Geometry check sheet. Reference: the model listing, model coordinates, mm. A direction names the side the tool comes from. Round coordinates to 2 decimals unless told otherwise and drop trailing zeros. Order: outer loops, then holes, each group sorted by start corner. A loop starts at its lowest first (then second) coordinate and runs counter-clockwise, first axis right, second up. Notation, with made-up numbers: (-6.5, 13.25) - (9.5, 13.25) arc R16 cw to (9.5, 27.25) - close; hole circle Ø4 at (53, 61). An arc over 180 degrees is marked (long way). Use a Markdown table: item, result. Add a question column.
(1) Section check D-D on z = 16. Record the boundary of the cut face in (x, y), then the cut area to 3 significant figures.
(2) Mould release check, pull along X, two halves, no side actions. Record for faces 1 (the face through (0.061, -17.445, 87.468)), 2 (the face through (0, 0, 126)), 3 (the face through (-10.88, -11.27, 87.47)): released by +X, released by -X, zero draft, split by the parting line, or undercut.
(3) Thickness scan on line 1 along X through (y, z) = (10.5, 53); line 2 along X through (y, z) = (14, 100); line 3 along Y through (x, z) = (-14.5, 103.5). Record the ranges inside material, lowest first. Write a range as [from, to].
(4) Section check B-B on y = 0. Record the boundary of the cut face in (x, z) (3 decimals).
(5) Gauge pin test, flat ends, axial feed: P1, Ø6, axis at y = 12, z = 88, coming from the -X side; P2, Ø12, axis at x = 9, z = 33, coming from the +Y side; P3, Ø10, axis at y = 1.5, z = 24.5, coming from the +X side. Record the tip position at first contact, or that the pin passes through.
(6) Access from +Z, -Z, +X, -X, +Y, -Y to the whole of each face (thin tool, end or side, straight path). Record for faces 4 (the face through (-10.922, 11.294, 87.468)), 5 (the face through (15.198, -3.786, 87.468)), 6 (the face through (-5, -12, 50)).
(7) Section check A-A on x = 0. Record the boundary of the cut face in (y, z) (3 decimals).
(8) Section check C-C on z = 59.5. Record the boundary of the cut face in (x, y) (3 decimals), then the cut area to 3 significant figures.
```python
from build123d import *

# Parameters (mm, degrees)
SKETCH1_R           = 12.5
BOSS_EXTRUDE1_DEPTH = 50
BOSS_EXTRUDE2_DEPTH = 76


with BuildPart() as part:
    # Sketch1 → Boss-Extrude1 (new body)
    with BuildSketch(Plane.XY):
        Circle(SKETCH1_R)
    extrude(amount=BOSS_EXTRUDE1_DEPTH)

    # Sketch2 → Boss-Extrude2 (add)
    with BuildSketch(Plane.XY.offset(50)):
        with BuildLine():
            Line((9.322615937, 10.370721146), (12.477254481, 12.192052559))
            ThreePointArc((12.477254481, 12.192052559), (15.107813169, 8.7225), (16.797254481, 4.709593071))
            Line((16.797254481, 4.709593071), (13.642615937, 2.888261658))
            ThreePointArc((13.642615937, 2.888261658), (13.945, 0), (13.642615937, -2.888261658))
            Line((13.642615937, -2.888261658), (16.797254481, -4.709593071))
            ThreePointArc((16.797254481, -4.709593071), (15.107813169, -8.7225), (12.477254481, -12.192052559))
            Line((12.477254481, -12.192052559), (9.322615937, -10.370721146))
            ThreePointArc((9.322615937, -10.370721146), (6.9725, -12.076724256), (4.32, -13.258982804))
            Line((4.32, -13.258982804), (4.32, -16.90164563))
            ThreePointArc((4.32, -16.90164563), (0, -17.445), (-4.32, -16.90164563))
            Line((-4.32, -16.90164563), (-4.32, -13.258982804))
            ThreePointArc((-4.32, -13.258982804), (-6.9725, -12.076724256), (-9.322615937, -10.370721146))
            Line((-9.322615937, -10.370721146), (-12.477254481, -12.192052559))
            ThreePointArc((-12.477254481, -12.192052559), (-15.107813169, -8.7225), (-16.797254481, -4.709593071))
            Line((-16.797254481, -4.709593071), (-13.642615937, -2.888261658))
            ThreePointArc((-13.642615937, -2.888261658), (-13.945, 0), (-13.642615937, 2.888261658))
            Line((-13.642615937, 2.888261658), (-16.797254481, 4.709593071))
            ThreePointArc((-16.797254481, 4.709593071), (-15.107813169, 8.7225), (-12.477254481, 12.192052559))
            Line((-12.477254481, 12.192052559), (-9.322615937, 10.370721146))
            ThreePointArc((-9.322615937, 10.370721146), (-6.9725, 12.076724256), (-4.32, 13.258982804))
            Line((-4.32, 13.258982804), (-4.32, 16.90164563))
            ThreePointArc((-4.32, 16.90164563), (0, 17.445), (4.32, 16.90164563))
            Line((4.32, 16.90164563), (4.32, 13.258982804))
            ThreePointArc((4.32, 13.258982804), (6.9725, 12.076724256), (9.322615937, 10.370721146))
        make_face()
    extrude(amount=BOSS_EXTRUDE2_DEPTH)


solid = part.part
```
Check sheet entries:
| question | item | result |
|---|---|---|
| 1 | outline | circle Ø25 at (0, 0) |
| 1 | area | 491 mm2 |
| 2 | face 1 | split by the parting line |
| 2 | face 2 | zero draft |
| 2 | face 3 | undercut |
| 3 | line 1 | x = [-13.93, -9.55], [-9.18, 9.18], [9.55, 13.93] |
| 3 | line 2 | x = [-4.32, 4.32] |
| 3 | line 3 | y = [-9.7, -3.38], [3.38, 9.7] |
| 4 | outline | (-13.945, 50) - (-12.5, 50) - (-12.5, 0) - (12.5, 0) - (12.5, 50) - (13.945, 50) - (13.945, 126) - (-13.945, 126) - close |
| 5 | P1 | stops at x = -14.94 |
| 5 | P2 | stops at y = 12.13 |
| 5 | P3 | stops at x = 12.5 |
| 6 | face 4 | +Z, -Z, +Y |
| 6 | face 5 | +Z, -Z, +X |
| 6 | face 6 | -Z |
| 7 | outline | (-17.445, 50) - (-12.5, 50) - (-12.5, 0) - (12.5, 0) - (12.5, 50) - (17.445, 50) - (17.445, 126) - (-17.445, 126) - close |
| 8 | outline | (-16.797, -4.71) arc R17.445 ccw to (-12.477, -12.192) - (-9.323, -10.371) arc R13.945 ccw to (-4.32, -13.259) - (-4.32, -16.902) arc R17.445 ccw to (4.32, -16.902) - (4.32, -13.259) arc R13.945 ccw to (9.323, -10.371) - (12.477, -12.192) arc R17.445 ccw to (16.797, -4.71) - (13.643, -2.888) arc R13.945 ccw to (13.643, 2.888) - (16.797, 4.71) arc R17.445 ccw to (12.477, 12.192) - (9.323, 10.371) arc R13.945 ccw to (4.32, 13.259) - (4.32, 16.902) arc R17.445 ccw to (-4.32, 16.902) - (-4.32, 13.259) arc R13.945 ccw to (-9.323, 10.371) - (-12.477, 12.192) arc R17.445 ccw to (-16.797, 4.71) - (-13.643, 2.888) arc R13.945 ccw to (-13.643, -2.888) - close |
| 8 | area | 795 mm2 |
